Geometry check sheet. Reference: the model listing, model coordinates, mm. Face numbers are marked on the shaded views. A direction names the side the tool comes from. Round coordinates to 2 decimals unless told otherwise and drop trailing zeros. Loops run counter-clockwise (first coordinate to the right, second up) from the corner with the lowest first, then second, coordinate; pieces in that order, holes last. Notation, with made-up numbers: (49.5, -36.5) -> (107.5, -36.5) arc R15 ccw to (107.5, -22.5) -> close; hole circle Ø5 at (5.5, -35). An arc over 180 degrees is marked (long way). Use a Markdown table: item, result. Add a question column.
Q1. Gauge pin test, flat ends, axial feed: P1, Ø0.9, axis at x = 0, y = 12.15, coming from the +Z side; P2, Ø3, axis at x = 0, y = 6.5, coming from the -Z side; P3, Ø3, axis at y = 8, z = 1, coming from the -X side. Record the tip position at first contact, or that the pin passes through.
Q2. Release check for a two-part mould opening along X. For the marked faces 3, 4 and 5 record: released by +X, released by -X, zero draft, split by the parting line, or undercut.
Q3. Sectioned sample at B-B, the plane y = 12.15. Enter the section's corners in (x, z).
Q4. Material ranges on L1, parallel to Y at x = 0, z = 0.1; L2, parallel to X at y = 12.15, z = 0.1; L3, parallel to Z at x = 0, y = 4.75, recorded low to high.
Q5. Sectioned sample at A-A, the plane z = 0. Enter the section's corners in (x, y).
Q6. Sectioned sample at C-C, the plane x = -1. Enter the section's corners in (y, z), then the cut area to 3 significant figures.
Q7. Set-up check for the marked faces 1 and 2: record each of +Z, -Z, +X, -X, +Y, -Y from which the full face is reachable in a straight line by a thin tool's end or side.
Q8. Sectioned sample at D-D, the plane y = 4.75. Enter the section's corners in (x, z), then the cut area to 3 significant figures.
```python
from build123d import *

# Parameters (mm, degrees)
SKETCH2_R               = 3.1
BOSS_EXTRUDE1_DEPTH     = 2.5
SKETCH3_R               = 1.8
BOSS_EXTRUDE3_DEPTH     = 11
CUT_EXTRUDE1_DEPTH      = 15.194012822
CUT_EXTRUDE1_DEPTH_BACK = 15.194012822
SKETCH4_R               = 0.75


with BuildPart() as part:
    # Sketch2 → Boss-Extrude1 (new body)
    with BuildSketch(Plane(origin=(0, 0, 0), x_dir=(1, 0, 0), z_dir=(0, 1, 0))):
        with Locations(Location((0, 0, 0), (0, 0, 270))):
            Circle(SKETCH2_R)
    extrude(amount=BOSS_EXTRUDE1_DEPTH)

    # Sketch3 → Boss-Extrude3 (add)
    with BuildSketch(Plane(origin=(0, 2.5, 0), x_dir=(1, 0, 0), z_dir=(0, 1, 0))):
        with Locations(Location((0, 0, 0), (0, 0, 270))):
            Circle(SKETCH3_R)
    extrude(amount=BOSS_EXTRUDE3_DEPTH)

    # Sketch4 → Cut-Extrude1 (cut, two sides: drawn at the far end of the back side and taken through both)
    with BuildSketch(Plane.XY.offset(-CUT_EXTRUDE1_DEPTH_BACK)):
        with Locations(Location((0, 12.15, 0), (0, 0, 90))):
            Circle(SKETCH4_R)
    extrude(amount=CUT_EXTRUDE1_DEPTH + CUT_EXTRUDE1_DEPTH_BACK, mode=Mode.SUBTRACT)


solid = part.part
```
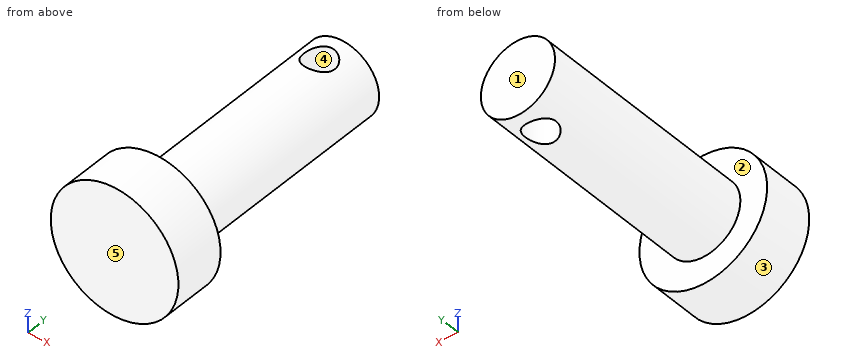
Values:
| question | item | result |
|---|---|---|
| 1 | P1 | through |
| 1 | P2 | z = -1.8 |
| 1 | P3 | x = -1.8 |
| 2 | face 3 | split by the parting line |
| 2 | face 4 | undercut |
| 2 | face 5 | zero draft |
| 3 | outline | (-0.75, -1.64) -> (-0.75, 1.64) arc R1.8 ccw to start; (0.75, -1.64) arc R1.8 ccw to (0.75, 1.64) -> close |
| 4 | L1 | 0 to 11.4, 12.9 to 13.5 |
| 4 | L2 | -1.8 to -0.75, 0.75 to 1.8 |
| 4 | L3 | -1.8 to 1.8 |
| 5 | outline | (-3.1, 0) -> (3.1, 0) -> (3.1, 2.5) -> (1.8, 2.5) -> (1.8, 13.5) -> (-1.8, 13.5) -> (-1.8, 2.5) -> (-3.1, 2.5) -> close; hole circle Ø1.5 at (0, 12.15) |
| 6 | outline | (0, -2.93) -> (2.5, -2.93) -> (2.5, -1.5) -> (13.5, -1.5) -> (13.5, 1.5) -> (2.5, 1.5) -> (2.5, 2.93) -> (0, 2.93) -> close |
| 6 | area | 47.6 mm^2 |
| 7 | face 1 | +Z, -Z, +X, -X, +Y |
| 7 | face 2 | +Y |
| 8 | outline | circle Ø3.6 at (0, 0) |
| 8 | area | 10.2 mm^2 |
